```python
from build123d import *

# Parameters (mm, degrees)
CONE006_ANGLE           = 28
CONE003_ANGLE           = 24
CONE003_PLACEMENT_ANGLE = 1.999999
CONE002_ANGLE           = 28
POCKET_DEPTH            = 5


with BuildPart() as obj1:
    # Cone006 → Cone006 (revolve)
    with BuildSketch(Plane(origin=(0, 0, 12), x_dir=(1, 0, 0), z_dir=(0, -1, 0))):
        Polygon((0, 0), (20, 0), (27, 40), (0, 40), align=None)
    revolve(axis=Axis((0, 0, 12), (0, 0, 1)), revolution_arc=CONE006_ANGLE)


with BuildPart() as obj2:
    # Cone003 → Cone003 (revolve)
    with BuildSketch(Plane.XZ):
        Polygon((0, 0), (36.5, 0), (43.5, 39), (0, 39), align=None)
    revolve(axis=Axis((0, 0, 0), (0, 0, 1)), revolution_arc=CONE003_ANGLE)


with BuildPart() as obj2_1:
    # Cone003 placement: moved
    add(obj2.part.moved(Location((0, 0, 13))).rotate(Axis((0, 0, 13), (0, 0, 1)), CONE003_PLACEMENT_ANGLE))


with BuildPart() as obj3:
    # Cone002 → Cone002 (revolve)
    with BuildSketch(Plane(origin=(0, 0, 12), x_dir=(1, 0, 0), z_dir=(0, -1, 0))):
        Polygon((0, 0), (38, 0), (45, 40), (0, 40), align=None)
    revolve(axis=Axis((0, 0, 12), (0, 0, 1)), revolution_arc=CONE002_ANGLE)

    # Cut001: cut obj2
    add(obj2_1.part, mode=Mode.SUBTRACT)

    # Cut003: cut obj1
    add(obj1.part, mode=Mode.SUBTRACT)

    # Sketch011 → Pocket (cut)
    with BuildSketch(Plane(origin=(0, 0, 12), x_dir=(1, 0, 0), z_dir=(0, 0, -1))):
        with BuildLine():
            ThreePointArc((20.103216, -8.936482), (21.348889, -5.312713), (21.946889, -1.527769))
            Line((21.946889, -1.527769), (23.94206, -1.666658))
            ThreePointArc((21.930781, -9.748889), (23.289698, -5.795687), (23.94206, -1.666658))
            Line((20.103216, -8.936482), (21.930781, -9.748889))
        make_face()
        with BuildLine():
            ThreePointArc((23.758346, -10.561297), (25.230506, -6.278661), (25.937232, -1.805546))
            Line((25.937232, -1.805546), (27.932594, -1.944447))
            ThreePointArc((25.586086, -11.373782), (27.171499, -6.761681), (27.932594, -1.944447))
            Line((23.758346, -10.561297), (25.586086, -11.373782))
        make_face()
        with BuildLine():
            ThreePointArc((27.413476, -12.186112), (29.112122, -7.244609), (29.927575, -2.083322))
            Line((29.927575, -2.083322), (31.922747, -2.22221))
            ThreePointArc((29.241041, -12.998519), (31.05293, -7.727583), (31.922747, -2.22221))
            Line((27.413476, -12.186112), (29.241041, -12.998519))
        make_face()
        with BuildLine():
            ThreePointArc((31.068797, -13.811011), (32.993941, -8.210607), (33.918127, -2.361113))
            Line((33.918127, -2.361113), (35.913287, -2.5))
            ThreePointArc((32.896352, -14.623414), (34.934737, -8.693578), (35.913287, -2.5))
            Line((31.068797, -13.811011), (32.896352, -14.623414))
        make_face()
    extrude(amount=-POCKET_DEPTH, mode=Mode.SUBTRACT)


solid = obj3.part
```
Model file for the job. Use its own axes, mm. A direction names the side the tool comes from. Coordinates: 2 decimals unless noted, no trailing zeros. Write each loop counter-clockwise with the first axis right and the second up, starting at its lowest first coordinate (ties: lowest second). Pieces come first, ordered by that corner, then holes. Notation, with made-up numbers: (37.5, 10.5) - (92.5, 10.5) arc R34 cw to (92.5, 42.5) - close; hole circle Ø2 at (16.5, 66). An arc over 180 degrees is marked (long way). Use a Markdown table: item, result. Add a question column.
Item 1: Band-saw the part on A-A, the plane z = 42. Write the cut outline in (x, y).
Item 2: Two-plate mould, pull along X, no slides. Class faces 4 (the face through (22.73, 0.59, 27.65)), 5 (the face through (31.034, 7.803, 12.493)), 6 (the face through (42.2, 11.4, 52)), 7 (the face through (31.97, 14.21, 12.49)): pulls with the +X half, pulls with the -X half, needs draft (parallel to the pull), parting line crosses it, or undercut.
Item 3: 3-axis set-ups, long thin cutter, end or side, ignore diameter. For faces 1 (the face through (32, 0, 32)), 2 (the face through (27.4, 6.8, 13)), 3 (the face through (24.66, 10.96, 12.49)): which of +Z, -Z, +X, -X, +Y, -Y reach the whole face in a straight line?
Item 4: Drop flat-ended pins along their axis: pin 1 (1 mm diameter, centred on y = 13.5, z = 32, fed in from -X); pin 2 (10 mm diameter, centred on x = 31, y = 13, fed in from +Z); pin 3 (1 mm diameter, centred on x = 22, y = 9.5, fed in from +Z); pin 4 (6 mm diameter, centred on x = 25, z = 36.5, fed in from +Y). Give the stop position or say it passes through.
Item 5: Band-saw the part on C-C, the plane z = 49. Write the cut outline in (x, y) (3 decimals), and give its area (3 significant figures).
Item 6: Band-saw the part on B-B, the plane y = 6.5. Give the number of separate pieces and of enclosed holes in the cut face, and give its area (3 significant figures).
Item 7: Drill centre lines: line 1 along Z through (x, y) = (26, 12.5); line 2 along Y through (x, z) = (32.75, 19); line 3 along Y through (x, z) = (21, 16). Where is each one in solid material? Low to high.
A:
| question | item | result |
|---|---|---|
| 1 | outline | (22.29, 11.85) arc R25.25 cw to (22.69, 11.07) - (37.48, 18.28) arc R41.71 cw to (41.68, 1.46) - (25.23, 0.88) arc R25.25 cw to (25.25, 0) - (43.25, 0) arc R43.25 ccw to (38.19, 20.3) - close |
| 2 | face 4 | pulls with the -X half |
| 2 | face 5 | undercut |
| 2 | face 6 | needs draft |
| 2 | face 7 | undercut |
| 3 | face 1 | +Z, -Z, +X, -X, -Y |
| 3 | face 2 | +Z |
| 3 | face 3 | +Z, -Z |
| 4 | pin 1 | stops at x = 24.45 |
| 4 | pin 2 | stops at z = 52 |
| 4 | pin 3 | stops at z = 13 |
| 4 | pin 4 | stops at y = 14.89 |
| 5 | outline | (23.376, 12.429) arc R26.475 cw to (23.796, 11.606) - (38.614, 18.833) arc R42.962 cw to (42.935, 1.499) - (26.459, 0.924) arc R26.475 cw to (26.475, 0) - (44.475, 0) arc R44.475 ccw to (39.269, 20.88) - close |
| 5 | area | 72.3 mm² |
| 6 | separate pieces | 5 |
| 6 | enclosed holes | 0 |
| 6 | area | 73.0 mm² |
| 7 | line 1 | z = 12 to 13 |
| 7 | line 2 | y = 0 to 1.14, 15.97 to 17.41 |
| 7 | line 3 | y = 0 to 0.73, 10.24 to 11.17 |
